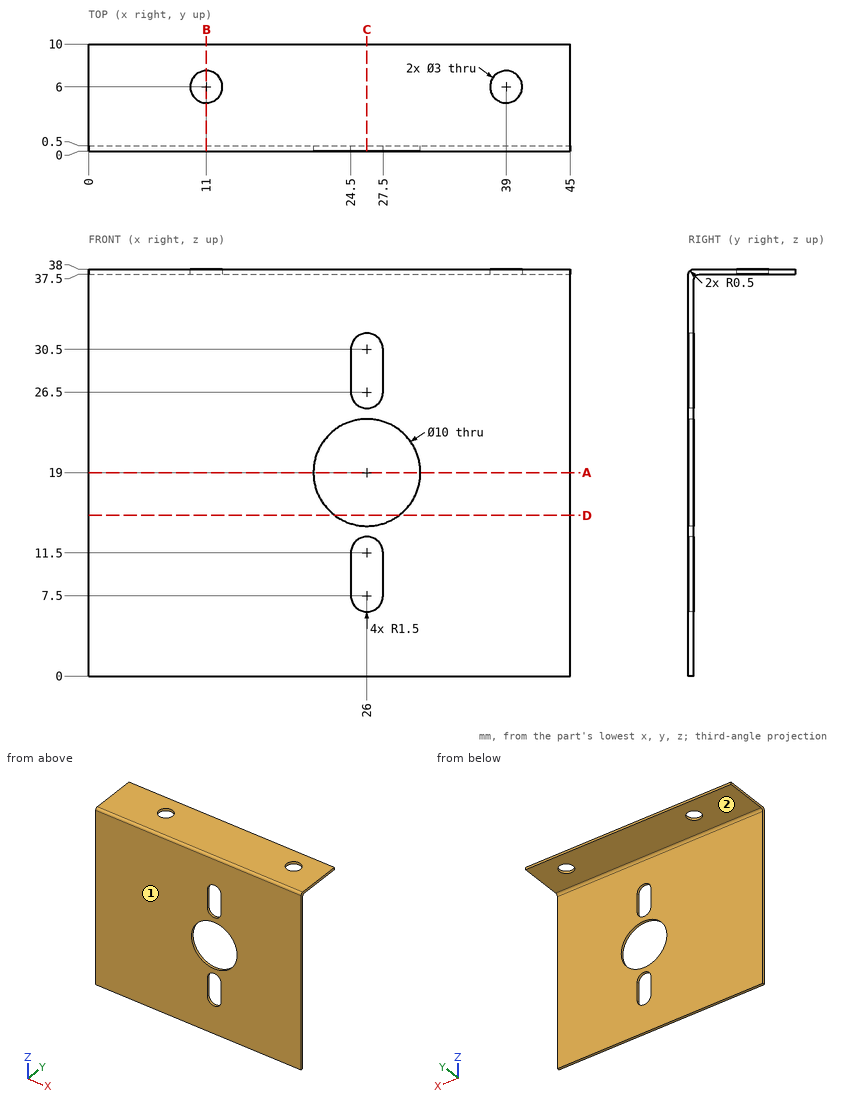
Design review of the part shown in the three views and the two pictorial views. Dimensions are in mm from the part's minimum x, y and z. A direction names the side the tool comes from. Round coordinates to 2 decimals unless told otherwise and drop trailing zeros. Loops run counter-clockwise (first coordinate to the right, second up) from the corner with the lowest first, then second, coordinate; pieces in that order, holes last. Notation, with made-up numbers: M 64,81.5 L 95,81.5 A20 ccw 95,91.5 Z; hole C 18,-11 d10. An arc over 180 degrees is marked long. Answer as a JSON object with one key per item and string values.
Item 1: We need section D-D, the plane z = 15. State the section outline as (x, y) points.
Check sheet entries:
{"outline": "M 0,0 L 23,0 L 23,0.5 L 0,0.5 Z; M 29,0 L 45,0 L 45,0.5 L 29,0.5 Z"}
Item 2: We need section A-A, the plane z = 19. State the section outline as (x, y) points.
Check sheet entries:
{"outline": "M 0,0 L 21,0 L 21,0.5 L 0,0.5 Z; M 31,0 L 45,0 L 45,0.5 L 31,0.5 Z"}
Item 3: We need section B-B, the plane x = 11. State the section outline as (y, z) points, and give its area (4 significant figures).
Check sheet entries:
{"outline": "M 0,0 L 0.5,0 L 0.5,37 A0.5 cw 1,37.5 L 4.5,37.5 L 4.5,38 L 0.5,38 A0.5 ccw 0,37.5 Z; M 7.5,37.5 L 10,37.5 L 10,38 L 7.5,38 Z", "area": "22.25 mm2"}
Item 4: Clearance check with flat-ended pins moving along their axes: P1, Ø5, axis at x = 9, y = 5, coming from the -Z side; P2, Ø3, axis at y = 2.5, z = 9.5, coming from the +X side. State where each tip first meets the part, or that it passes through.
Check sheet entries:
{"P1": "z = 37.5", "P2": "through"}
Item 5: For line 1 along Y through (x, z) = (11, 37.6); line 2 along Z through (x, y) = (26, 0.35); line 3 along Z through (x, y) = (42, 5.5), list the stretches that pass through material, from the lowest coordinate up.
Check sheet entries:
{"line 1": "0.01 to 4.5, 7.5 to 10", "line 2": "0 to 6, 13 to 14, 24 to 25, 32 to 37.98", "line 3": "37.5 to 38"}
Item 6: We need section C-C, the plane x = 26. State the section outline as (y, z) points, and give its area (4 significant figures).
Check sheet entries:
{"outline": "M 0,0 L 0.5,0 L 0.5,6 L 0,6 Z; M 0,13 L 0.5,13 L 0.5,14 L 0,14 Z; M 0,24 L 0.5,24 L 0.5,25 L 0,25 Z; M 0,32 L 0.5,32 L 0.5,37 A0.5 cw 1,37.5 L 10,37.5 L 10,38 L 0.5,38 A0.5 ccw 0,37.5 Z", "area": "11.75 mm2"}
Item 7: Tool access review of the marked faces 1 and 2: name each direction out of +Z, -Z, +X, -X, +Y, -Y from which nothing blocks a thin tool from reaching the whole face with its end or side.
Check sheet entries:
{"face 1": "+Z, -Z, +X, -X, -Y", "face 2": "-Z, +X, -X, +Y"}
